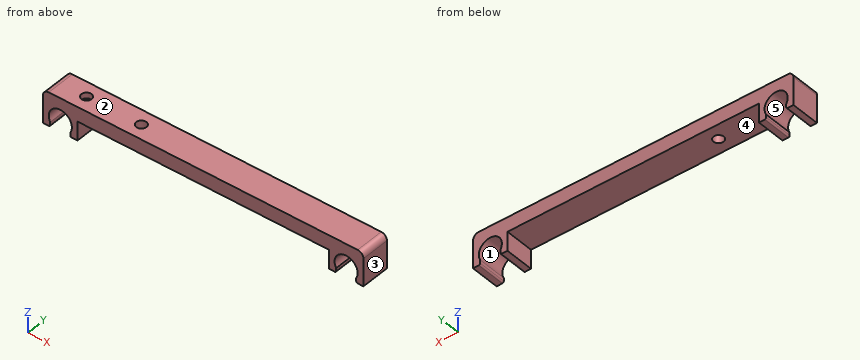
```python
from build123d import *

# Parameters (mm, degrees)
BOSS_EXTRUDE1_DEPTH = 10
FILLET1_R           = 2
FILLET2_R           = 2
FILLET3_R           = 0.5
FILLET4_R           = 0.5
FILLET5_R           = 0.5
FILLET6_R           = 0.5
MOUNTING_HOLE_R     = 1.75
CUT_EXTRUDE1_DEPTH  = 5
MOUNTING_CONE_R     = 1.75
CUT_EXTRUDE2_DEPTH  = 2


with BuildPart() as part:
    # Clip → Boss-Extrude1 (new body)
    with BuildSketch(Plane(origin=(0, 0, 0), x_dir=(1, 0, 0), z_dir=(0, 1, 0))):
        with BuildLine():
            Line((-55.5, 0), (55.5, 0))
            Line((55.5, 0), (55.5, 11.536491673))
            Line((55.5, 11.536491673), (53, 11.536491673))
            Line((53, 11.536491673), (53, 9.936491673))
            ThreePointArc((53, 9.936491673), (49.442392127, 4.000414855), (46.057224715, 10.036491673))
            Line((46.057224715, 10.036491673), (46.057224715, 11.536491673))
            Line((46.057224715, 11.536491673), (43.557224715, 11.536491673))
            Line((43.557224715, 11.536491673), (43.557224715, 5))
            Line((43.557224715, 5), (-43.557224715, 5))
            Line((-43.557224715, 5), (-43.557224715, 11.536491673))
            Line((-43.557224715, 11.536491673), (-46.057224715, 11.536491673))
            Line((-46.057224715, 11.536491673), (-46.057224715, 10.036491673))
            ThreePointArc((-46.057224715, 10.036491673), (-49.442392127, 4.000414855), (-53, 9.936491673))
            Line((-53, 9.936491673), (-53, 11.536491673))
            Line((-53, 11.536491673), (-55.5, 11.536491673))
            Line((-55.5, 11.536491673), (-55.5, 0))
        make_face()
    extrude(amount=BOSS_EXTRUDE1_DEPTH)

    # Fillet1
    fillet1_edges = [part.edges().sort_by_distance(p)[0] for p in [
        (55.5, 5, 0),
    ]]
    fillet(fillet1_edges, radius=FILLET1_R)

    # Fillet2
    fillet2_edges = [part.edges().sort_by_distance(p)[0] for p in [
        (-55.5, 5, 0),
    ]]
    fillet(fillet2_edges, radius=FILLET2_R)

    # Fillet3
    fillet3_edges = [part.edges().sort_by_distance(p)[0] for p in [
        (46.057224715, 5, -11.536491673),
    ]]
    fillet(fillet3_edges, radius=FILLET3_R)

    # Fillet4
    fillet4_edges = [part.edges().sort_by_distance(p)[0] for p in [
        (53, 5, -11.536491673),
    ]]
    fillet(fillet4_edges, radius=FILLET4_R)

    # Fillet5
    fillet5_edges = [part.edges().sort_by_distance(p)[0] for p in [
        (-53, 5, -11.536491673),
    ]]
    fillet(fillet5_edges, radius=FILLET5_R)

    # Fillet6
    fillet6_edges = [part.edges().sort_by_distance(p)[0] for p in [
        (-46.057224715, 5, -11.536491673),
    ]]
    fillet(fillet6_edges, radius=FILLET6_R)

    # Mounting Hole → Cut-Extrude1 (cut)
    with BuildSketch(Plane.XY):
        with Locations((-25.5, 5)):
            Circle(MOUNTING_HOLE_R)
    extrude(amount=-CUT_EXTRUDE1_DEPTH, mode=Mode.SUBTRACT)

    # Mounting Cone → Cut-Extrude2 (cut)
    with BuildSketch(Plane.XY):
        with Locations((-44.5, 5)):
            Circle(MOUNTING_CONE_R)
    extrude(amount=-CUT_EXTRUDE2_DEPTH, mode=Mode.SUBTRACT)


solid = part.part
```
Design review of the part built by this model. Coordinates are the model's own, in mm. Face numbers are marked on the shaded views. A direction names the side the tool comes from. Coordinates: 2 decimals unless noted, no trailing zeros. Write each loop counter-clockwise with the first axis right and the second up, starting at its lowest first coordinate (ties: lowest second). Pieces come first, ordered by that corner, then holes. Notation, with made-up numbers: M 27.5,-13.5 L 36.5,-13.5 A22 ccw 36.5,10.5 Z; hole C 19.5,-7 d1. An arc over 180 degrees is marked long. Answer as a JSON object with one key per item and string values.
Item 1: Add section C-C, the plane y = 9. Give the boundary of the cut face in (x, z), and give its area (3 significant figures).
Outcome:
{"outline": "M -55.5,-11.54 L -53.5,-11.54 A0.5 ccw -53,-11.04 L -53,-9.94 A4 cw long -46.06,-10.04 L -46.06,-11.04 A0.5 ccw -45.56,-11.54 L -43.56,-11.54 L -43.56,-5 L 43.56,-5 L 43.56,-11.54 L 45.56,-11.54 A0.5 ccw 46.06,-11.04 L 46.06,-10.04 A4 cw long 53,-9.94 L 53,-11.04 A0.5 ccw 53.5,-11.54 L 55.5,-11.54 L 55.5,-2 A2 ccw 53.5,0 L -53.5,0 A2 ccw -55.5,-2 Z", "area": "607 mm²"}
Item 2: Add section B-B, the plane z = -8. Give the boundary of the cut face in (x, y), and give its area (3 significant figures).
Outcome:
{"outline": "M -55.5,0 L -53.5,0 L -53.5,10 L -55.5,10 Z; M -45.5,0 L -43.56,0 L -43.56,10 L -45.5,10 Z; M 43.56,0 L 45.5,0 L 45.5,10 L 43.56,10 Z; M 53.5,0 L 55.5,0 L 55.5,10 L 53.5,10 Z", "area": "78.9 mm²"}
Item 3: Insertion check: pin 1 Ø1 at (x, y) = (-7.5, 3) entering from -Z. The pin has a flat end and moves straight along its axis. Give the tip position at first contact, or say it passes through.
Outcome:
{"pin 1": "z = -5"}
Item 4: Add section D-D, the plane x = 28. Give the boundary of the cut face in (y, z).
Outcome:
{"outline": "M 0,-5 L 10,-5 L 10,0 L 0,0 Z"}
Item 5: Wall thickness on probe 1 along X at (y, z) = (5, -6); probe 2 along X at (y, z) = (3.5, -1.5); probe 3 along X at (y, z) = (0.75, -7): over which ranges is each line inside the solid? List them lowest first.
Outcome:
{"probe 1": "-55.5 to -52.96, -46.04 to -43.56, 43.56 to 46.04, 52.96 to 55.5", "probe 2": "-55.44 to -45.4, -43.6 to -26.4, -24.6 to 55.44", "probe 3": "-55.5 to -53.37, -45.63 to -43.56, 43.56 to 45.63, 53.37 to 55.5"}
Item 6: Machinability: for the marked faces 4 and 5, which of the approach directions +Z, -Z, +X, -X, +Y, -Y give a long, thin tool a straight path to every point of the face, cutting with its end or side? Answer none if there is none.
Outcome:
{"face 4": "-Z, +Y, -Y", "face 5": "+Y, -Y"}
Item 7: Draft analysis for pull direction X (two halves, no side actions). For the marked faces 1, 2 and 3, state which applies: pulls with the +X half, pulls with the -X half, needs draft (parallel to the pull), parting line crosses it, or undercut.
Outcome:
{"face 1": "undercut", "face 2": "needs draft", "face 3": "pulls with the +X half"}
